The listing builds one solid part. Answer for the finished solid, in the listing's coordinates (mm). Face numbers are marked on the shaded views. Coordinates: 2 decimals unless noted, no trailing zeros. Order: outer loops, then holes, each group sorted by start corner. A loop starts at its lowest first (then second) coordinate and runs counter-clockwise, first axis right, second up. Notation, with made-up numbers: (72, 54.5) -> (120, 54.5) arc R23 cw to (120, 68.5) -> close; hole circle Ø3 at (27, 14.5). An arc over 180 degrees is marked (long way). Write item = value, one per line. Start each with the question number.
```python
from build123d import *

# Parameters (mm, degrees)
SKETCH1_W                       = 50.8
SKETCH1_H                       = 12.7
BOSS_EXTRUDE1_DEPTH             = 6.35
TAP_DRILL_FOR_1_4_20_TAP1_D     = 5.1054
TAP_DRILL_FOR_1_4_20_TAP1_DEPTH = 6.35
FILLET1_R                       = 3.175


with BuildPart() as part:
    # Sketch1 → Boss-Extrude1 (new body)
    with BuildSketch(Plane(origin=(0, 0, 0), x_dir=(1, 0, 0), z_dir=(0, 1, 0))):
        with Locations((25.4, -6.35)):
            Rectangle(SKETCH1_W, SKETCH1_H)
    extrude(amount=BOSS_EXTRUDE1_DEPTH)

    # Tap Drill for 1/4-20 Tap1
    with Locations(Plane(origin=(0, 0, 0), x_dir=(-1, 0, 0), z_dir=(0, -1, 0))):
        with Locations((-9.525, -6.35), (-41.275, -6.35)):
            Hole(TAP_DRILL_FOR_1_4_20_TAP1_D / 2, depth=TAP_DRILL_FOR_1_4_20_TAP1_DEPTH)

    # Fillet1
    fillet1_edges = [part.edges().sort_by_distance(p)[0] for p in [
        (0, 3.175, 0),
        (50.8, 3.175, 0),
        (50.8, 3.175, 12.7),
        (0, 3.175, 12.7),
    ]]
    fillet(fillet1_edges, radius=FILLET1_R)


solid = part.part
```
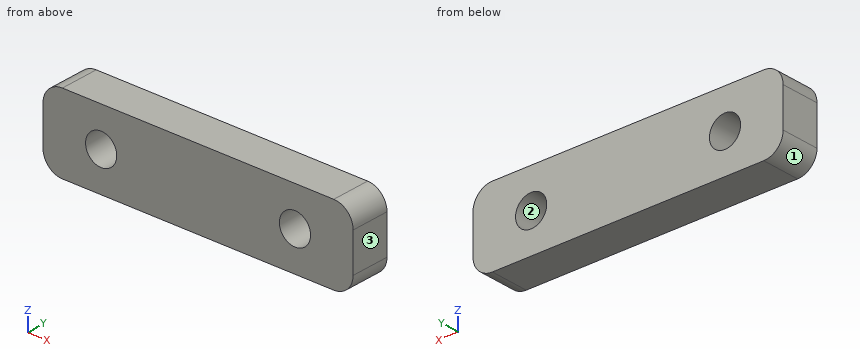
Item 1: Section C-C, the plane x = 9.5 is taken. Give the vertices of the cut face in (y, z), then the cut area to 3 significant figures.
Item 2: Section D-D, the plane z = 11.5 is taken. Give the vertices of the cut face in (x, y).
Item 3: Section B-B, the plane y = 4 is taken. Give the vertices of the cut face in (x, z) (3 decimals).
Item 4: Consider probe 1 along X at (y, z) = (5.75, 6); probe 2 along Z at (x, y) = (10, 2.25); probe 3 along Z at (x, y) = (8, 0.5). Determine where each line is inside the solid, lowest interval first.
Item 5: Section A-A, the plane z = 6.35 is taken. Give the vertices of the cut face in (x, y), then the cut area to 3 significant figures.
Item 6: For a pull along X with two mould halves and no side action, classify the marked faces 1, 2 and 3 as pulls with the +X half, pulls with the -X half, needs draft (parallel to the pull), parting line crosses it, or undercut.
A:
q1.outline = (0, 0) -> (6.35, 0) -> (6.35, 3.8) -> (0, 3.8) -> close; (0, 8.9) -> (6.35, 8.9) -> (6.35, 12.7) -> (0, 12.7) -> close
q1.area = 48.2 mm^2
q2.outline = (0.69, 0) -> (50.11, 0) -> (50.11, 6.35) -> (0.69, 6.35) -> close
q3.outline = (0, 3.175) arc R3.175 ccw to (3.175, 0) -> (47.625, 0) arc R3.175 ccw to (50.8, 3.175) -> (50.8, 9.525) arc R3.175 ccw to (47.625, 12.7) -> (3.175, 12.7) arc R3.175 ccw to (0, 9.525) -> close; hole circle Ø5.105 at (9.525, 6.35); hole circle Ø5.105 at (41.275, 6.35)
q4.probe_1 = 0 to 7, 12.05 to 38.75, 43.8 to 50.8
q4.probe_2 = 0 to 3.84, 8.86 to 12.7
q4.probe_3 = 0 to 4.3, 8.4 to 12.7
q5.outline = (0, 0) -> (6.97, 0) -> (6.97, 6.35) -> (0, 6.35) -> close; (12.08, 0) -> (38.72, 0) -> (38.72, 6.35) -> (12.08, 6.35) -> close; (43.83, 0) -> (50.8, 0) -> (50.8, 6.35) -> (43.83, 6.35) -> close
q5.area = 258 mm^2
q6.face_1 = pulls with the -X half
q6.face_2 = undercut
q6.face_3 = pulls with the +X half
